Model file for the job. Use its own axes, mm. A direction names the side the tool comes from. Coordinates: 2 decimals unless noted, no trailing zeros. Write each loop counter-clockwise with the first axis right and the second up, starting at its lowest first coordinate (ties: lowest second). Pieces come first, ordered by that corner, then holes. Notation, with made-up numbers: M 35,46.25 L 83,46.25 A20 ccw 83,74.25 Z; hole C -37,16 d7. An arc over 180 degrees is marked long. Put each result on its own line as item: value. Start each with the question number.
Q1. Pull direction Z, two halves, no side cores. Call faces 4 (the flat face through (95, 21, -14)), 5 (the flat face through (47, 0, -14)), 6 (the flat face through (47, 31, 0)): pulls with the +Z half, pulls with the -Z half, needs draft (parallel to the pull), parting line crosses it, or undercut.
Q2. Cut at B-B (x = 69). Write the cut outline in (y, z).
Q3. Drill centre lines: line 1 along Z through (x, y) = (86, 3); line 2 along X through (y, z) = (6.5, -2.75); line 3 along Y through (x, z) = (10.5, -6). Where is each one in solid material? Low to high.
Q4. Which spindle directions (+Z, -Z, +X, -X, +Y, -Y) get a long thin tool onto all of the face, cutting with end or side? Do faces 1 (the flat face through (95, 41, -18)), 2 (the flat face through (1, 15, -14)), 3 (the flat face through (46, 32, -26)). Say none if no direction does.
Q5. Cut at C-C (z = -16.5). Write the cut outline in (x, y), then the cut area to 3 significant figures.
Q6. Cut at A-A (y = 56.5). Write the cut outline in (x, z), then the cut area to 3 significant figures.
Q7. Drop flat-ended pins along their axis: pin 1 (2 mm diameter, centred on x = 95, z = -14.5, fed in from +Y); pin 2 (12 mm diameter, centred on x = 31, z = -8.5, fed in from +Y); pin 3 (5 mm diameter, centred on y = 43.5, z = -5.5, fed in from -X). Give the stop position or say it passes through.
```python
from build123d import *

# Parameters (mm, degrees)
SKETCH1_W           = 96
SKETCH1_H           = 28
BOSS_EXTRUDE1_DEPTH = 62
SKETCH2_W           = 92
SKETCH2_H           = 24
CUT_EXTRUDE1_DEPTH  = 60
SKETCH3_W           = 8
SKETCH3_H           = 41
CUT_EXTRUDE2_DEPTH  = 12
SKETCH4_W           = 24
SKETCH4_H           = 47
CUT_EXTRUDE3_DEPTH  = 10


with BuildPart() as part:
    # Sketch1 → Boss-Extrude1 (new body)
    with BuildSketch(Plane(origin=(0, 0, 0), x_dir=(1, 0, 0), z_dir=(0, 1, 0))):
        with Locations((48, 14)):
            Rectangle(SKETCH1_W, SKETCH1_H)
    extrude(amount=BOSS_EXTRUDE1_DEPTH)

    # Sketch2 → Cut-Extrude1 (cut)
    with BuildSketch(Plane(origin=(0, 62, 0), x_dir=(1, 0, 0), z_dir=(0, 1, 0))):
        with Locations((48, 14)):
            Rectangle(SKETCH2_W, SKETCH2_H)
    extrude(amount=-CUT_EXTRUDE1_DEPTH, mode=Mode.SUBTRACT)

    # Sketch3 → Cut-Extrude2 (cut)
    with BuildSketch(Plane(origin=(96, 0, 0), x_dir=(0, 0, -1), z_dir=(1, 0, 0))):
        with Locations((14, 41.5)):
            Rectangle(SKETCH3_W, SKETCH3_H)
    extrude(amount=-CUT_EXTRUDE2_DEPTH, mode=Mode.SUBTRACT)

    # Sketch4 → Cut-Extrude3 (cut)
    with BuildSketch(Plane.ZY):
        with Locations((-14, 38.5)):
            Rectangle(SKETCH4_W, SKETCH4_H)
    extrude(amount=-CUT_EXTRUDE3_DEPTH, mode=Mode.SUBTRACT)


solid = part.part
```
Computed values:
1. face 4: undercut
1. face 5: needs draft
1. face 6: pulls with the +Z half
2. outline: M 0,-28 L 62,-28 L 62,-26 L 2,-26 L 2,-2 L 62,-2 L 62,0 L 0,0 Z
3. line 1: -28 to -26, -2 to 0
3. line 2: 0 to 2, 94 to 96
3. line 3: 0 to 2
4. face 1: +X, -X, +Y
4. face 2: -X, +Y
4. face 3: +Y
5. outline: M 0,0 L 96,0 L 96,21 L 94,21 L 94,2 L 2,2 L 2,15 L 0,15 Z
5. area: 256 mm2
6. outline: M 0,-28 L 96,-28 L 96,-18 L 94,-18 L 94,-26 L 0,-26 Z; M 0,-2 L 94,-2 L 94,-10 L 96,-10 L 96,0 L 0,0 Z
6. area: 416 mm2
7. pin 1: y = 21
7. pin 2: y = 2
7. pin 3: x = 94
